from build123d import *

# Parameters (mm, degrees)
F0_R     = 3.75
F2_DEPTH = 25
F3_DEPTH = 14
F4_R     = 3.75
F6_DEPTH = 25
F7_DEPTH = 2.5


with BuildPart() as f2:
    # F0 (on Top) → F2 (new body)
    with BuildSketch(Plane.XY):
        with Locations((-20, 0)):
            Circle(F0_R)
        with Locations((20, 0)):
            Circle(F0_R)
    extrude(amount=F2_DEPTH)


with BuildPart() as f3:
    # F1 (on Top) → F3 (new body)
    with BuildSketch(Plane.XY):
        with BuildLine():
            ThreePointArc((-22.819472, 4.428666), (-22.525893, -4.60243), (-14.75, 0))
            ThreePointArc((-14.75, 0), (-17.474107, 4.60243), (-22.819472, 4.428666))
        make_face()
        with BuildLine():
            ThreePointArc((-22.819472, 4.428666), (-17.474107, 4.60243), (-14.75, 0))
            Line((-14.75, 0), (-7.5, 10.5))
            Line((-7.5, 10.5), (7.5, 10.5))
            Line((7.5, 10.5), (14.75, 0))
            ThreePointArc((14.75, 0), (17.377467, 4.548057), (22.629931, 4.543783))
            Line((22.629931, 4.543783), (10, 15.5))
            Line((10, 15.5), (-10, 15.5))
            Line((-10, 15.5), (-22.819472, 4.428666))
        make_face()
        with BuildLine():
            ThreePointArc((22.629931, 4.543783), (17.377467, 4.548057), (14.75, 0))
            ThreePointArc((14.75, 0), (20, -5.25), (25.25, 0))
            ThreePointArc((25.25, 0), (24.548057, 2.622533), (22.629931, 4.543783))
        make_face()
    extrude(amount=F3_DEPTH)


with BuildPart() as f6:
    # F4 (on face) → F6 (new body)
    with BuildSketch(Plane(origin=(0, 15.5, 0), x_dir=(-1, 0, 0), z_dir=(0, 1, 0))):
        with Locations((0, 8)):
            Circle(F4_R)
    extrude(amount=-F6_DEPTH)


with BuildPart() as f7:
    # F5 (on face) → F7 (new body)
    with BuildSketch(Plane.XZ.offset(-10.5)):
        Polygon((2.582829, 3.691985), (5.022265, 8.082788), (2.439436, 12.390803), (-2.582829, 12.308015), (-5.022265, 7.917212), (-2.439436, 3.609197), align=None)
    extrude(amount=-F7_DEPTH)


with BuildPart() as f3_1:
    add(f3.part)

    # F8: cut F2, F6, F7
    add(f2.part, mode=Mode.SUBTRACT)
    add(f6.part, mode=Mode.SUBTRACT)
    add(f7.part, mode=Mode.SUBTRACT)


solid = f3_1.part
Verification items for the finished model (mm, model axes). A direction names the side the tool comes from. Give positions to 0.01 mm unless a question says otherwise; leave off trailing zeros. Loops run counter-clockwise (first coordinate to the right, second up) from the corner with the lowest first, then second, coordinate; pieces in that order, holes last.
1. Release check for a two-part mould opening along Y. For faces 4 (the flat face through (3.749, 11.732, 10.207)), 5 (the flat face through (-11.176, 5.177, 6.902)), 6 (the cylindrical face through (-16.423, 1.126, 6.902)), 7 (the flat face through (16.4, 9.95, 6.9)) record: +Y half, -Y half, draft (parallel to the pull), parting line (faces both ways), or undercut.
Derived:
face 4: draft
face 5: -Y half
face 6: undercut
face 7: +Y half
2. Material ranges on probe 1 along X at (y, z) = (-0.25, 12.75); probe 2 along X at (y, z) = (-3, 9.5); probe 3 along Y at (x, z) = (20, 11), recorded low to high.
Derived:
probe 1: x = -25.24 to -23.74, -16.26 to -14.76, 14.76 to 16.26, 23.74 to 25.24
probe 2: x = -24.31 to -22.25, -17.75 to -15.69, 15.69 to 17.75, 22.25 to 24.31
probe 3: y = -5.25 to -3.75, 3.75 to 6.83
3. Go/stop test with flat-tipped pins: P1, Ø6, axis at x = 20, y = 0, coming from the +Z side; P2, Ø5, axis at y = 11, z = 10, coming from the +X side; P3, Ø2, axis at x = -19.5, z = 11.5, coming from the +Y side; P4, Ø8, axis at y = 10.5, z = 4, coming from the -X side. Record where each tip stops, or that it passes through.
Derived:
P1: passes through
P2: stops at x = 18.07
P3: stops at y = 8.16
P4: stops at x = -20.42
4. Tool access check on faces 1 (the flat face through (0, 15.5, 4)), 2 (the flat face through (-3.749, 11.732, 5.793)), 3 (the flat face through (11.074, 5.323, 6.902)). Record the directions out of +Z, -Z, +X, -X, +Y, -Y that give a thin tool (end or side, any length) a straight path to the whole face; none if there is none.
Derived:
face 1: +Z, -Z, +X, -X, +Y
face 2: -Y
face 3: +Z, -Z, -Y
5. Cross-section at B-B on x = 21.5. Record the cut outline in (y, z).
Derived:
outline: (-5.03, 0) - (-3.44, 0) - (-3.44, 14) - (-5.03, 14) - close; (3.44, 0) - (5.52, 0) - (5.52, 14) - (3.44, 14) - close
6. Cross-section at C-C on y = 6.5. Record the cut outline in (x, z).
Derived:
outline: (-20.42, 0) - (-10.26, 0) - (-10.26, 14) - (-20.42, 14) - close; (10.26, 0) - (20.37, 0) - (20.37, 14) - (10.26, 14) - close
7. Cross-section at D-D on z = 2.5. Record the cut outline in (x, y).
Derived:
outline: (-22.82, 4.43) arc R5.25 ccw (long way) to (-14.75, 0) - (-7.5, 10.5) - (7.5, 10.5) - (14.75, 0) arc R5.25 ccw (long way) to (22.63, 4.54) - (10, 15.5) - (-10, 15.5) - close; hole circle Ø7.5 at (-20, 0); hole circle Ø7.5 at (20, 0)
8. Cross-section at A-A on z = 9.5. Record the cut outline in (x, y).
Derived:
outline: (-22.82, 4.43) arc R5.25 ccw (long way) to (-14.75, 0) - (-7.5, 10.5) - (-4.14, 10.5) - (-4.14, 13) - (-3.44, 13) - (-3.44, 15.5) - (-10, 15.5) - close; (3.44, 13) - (4.17, 13) - (4.17, 10.5) - (7.5, 10.5) - (14.75, 0) arc R5.25 ccw (long way) to (22.63, 4.54) - (10, 15.5) - (3.44, 15.5) - close; hole circle Ø7.5 at (-20, 0); hole circle Ø7.5 at (20, 0)
